from build123d import *
from OCP.BRepFilletAPI import BRepFilletAPI_MakeChamfer

# Parameters (mm, degrees)
SKETCH1_W                = 0.64
SKETCH1_H                = 0.64
BOSS_EXTRUDE1_DEPTH      = 2.05
CUT_EXTRUDE1_DEPTH       = 5
SKETCH3_W                = 1.54
SKETCH3_H                = 0.5
BOSS_EXTRUDE2_DEPTH      = 0.5
BOSS_EXTRUDE3_DEPTH      = 10
BOSS_EXTRUDE3_DEPTH_BACK = 5.05
SKETCH4_W                = 0.64
SKETCH4_H                = 0.64
CHAMFER1_SIZE            = 0.2
CHAMFER1_SIZE2           = 0.115470054
SKETCH5_R                = 0.125
CUT_EXTRUDE2_DEPTH       = 1


with BuildPart() as part:
    # Sketch1 → Boss-Extrude1 (new body)
    with BuildSketch(Plane(origin=(0, 0, 0), x_dir=(1, 0, 0), z_dir=(0, 1, 0))):
        Polygon((-2.04, -1.27), (-0.5, -1.27), (0, -0.77), (0.5, -1.27), (2.04, -1.27), (2.54, -0.77), (2.54, 0.77), (2.04, 1.27), (0.5, 1.27), (0, 0.77), (-0.5, 1.27), (-2.04, 1.27), (-2.54, 0.77), (-2.54, -0.77), align=None)
        with Locations((1.27, 0)):
            Rectangle(SKETCH1_W, SKETCH1_H, mode=Mode.SUBTRACT)
        with Locations((-1.27, 0)):
            Rectangle(SKETCH1_W, SKETCH1_H, mode=Mode.SUBTRACT)
    extrude(amount=-BOSS_EXTRUDE1_DEPTH)

    # Sketch2 → Cut-Extrude1 (cut, symmetric)
    with BuildSketch(Plane.XY):
        Polygon((-2.54, -0.2), (-2.54, 0), (-2.34, 0), align=None)
        Polygon((-0.2, 0), (0.2, 0), (0, -0.2), align=None)
        Polygon((2.34, 0), (2.54, 0), (2.54, -0.2), align=None)
        Polygon((-2.54, -1.85), (-2.34, -2.05), (-2.54, -2.05), align=None)
        Polygon((-0.2, -2.05), (0, -1.85), (0.2, -2.05), align=None)
        Polygon((2.34, -2.05), (2.54, -1.85), (2.54, -2.05), align=None)
    extrude(amount=CUT_EXTRUDE1_DEPTH, both=True, mode=Mode.SUBTRACT)

    # Sketch3 → Boss-Extrude2 (add)
    with BuildSketch(Plane.XZ.offset(2.05)):
        with Locations((-1.27, -1.02)):
            Rectangle(SKETCH3_W, SKETCH3_H)
        with Locations((-1.27, 1.02)):
            Rectangle(SKETCH3_W, SKETCH3_H)
        with Locations((1.27, 1.02)):
            Rectangle(SKETCH3_W, SKETCH3_H)
        with Locations((1.27, -1.02)):
            Rectangle(SKETCH3_W, SKETCH3_H)
    extrude(amount=BOSS_EXTRUDE2_DEPTH)

    # Sketch4 → Boss-Extrude3 (add, two sides: drawn at the far end of the back side and taken through both)
    with BuildSketch(Plane(origin=(0, 0, 0), x_dir=(1, 0, 0), z_dir=(0, 1, 0)).offset(-BOSS_EXTRUDE3_DEPTH_BACK)):
        with Locations((-1.27, 0)):
            Rectangle(SKETCH4_W, SKETCH4_H)
        with Locations((1.27, 0)):
            Rectangle(SKETCH4_W, SKETCH4_H)
    extrude(amount=BOSS_EXTRUDE3_DEPTH + BOSS_EXTRUDE3_DEPTH_BACK)

    # Chamfer1: one chamfer whose edges measure the first distance from different faces: ONE call of the kernel's chamfer builder (chamfer() names one face for all edges)
    chamfer1_edges_1 = [part.edges().sort_by_distance(p)[0] for p in [
        (-1.59, -5.05, 0),
    ]]
    chamfer1_side_1 = [part.faces().sort_by_distance(p)[0] for p in [
        (-1.59, -3.55, 0),
    ]]
    chamfer1_edges_2 = [part.edges().sort_by_distance(p)[0] for p in [
        (-1.27, -5.05, -0.32),
    ]]
    chamfer1_side_2 = [part.faces().sort_by_distance(p)[0] for p in [
        (-1.27, -3.55, -0.32),
    ]]
    chamfer1_edges_3 = [part.edges().sort_by_distance(p)[0] for p in [
        (-0.95, -5.05, 0),
    ]]
    chamfer1_side_3 = [part.faces().sort_by_distance(p)[0] for p in [
        (-0.95, -3.55, 0),
    ]]
    chamfer1_edges_4 = [part.edges().sort_by_distance(p)[0] for p in [
        (-1.27, -5.05, 0.32),
    ]]
    chamfer1_side_4 = [part.faces().sort_by_distance(p)[0] for p in [
        (-1.27, -3.55, 0.32),
    ]]
    chamfer1_edges_5 = [part.edges().sort_by_distance(p)[0] for p in [
        (-1.59, 10, 0),
    ]]
    chamfer1_side_5 = [part.faces().sort_by_distance(p)[0] for p in [
        (-1.59, 5, 0),
    ]]
    chamfer1_edges_6 = [part.edges().sort_by_distance(p)[0] for p in [
        (-1.27, 10, 0.32),
    ]]
    chamfer1_side_6 = [part.faces().sort_by_distance(p)[0] for p in [
        (-1.27, 5, 0.32),
    ]]
    chamfer1_edges_7 = [part.edges().sort_by_distance(p)[0] for p in [
        (-0.95, 10, 0),
    ]]
    chamfer1_side_7 = [part.faces().sort_by_distance(p)[0] for p in [
        (-0.95, 5, 0),
    ]]
    chamfer1_edges_8 = [part.edges().sort_by_distance(p)[0] for p in [
        (-1.27, 10, -0.32),
    ]]
    chamfer1_side_8 = [part.faces().sort_by_distance(p)[0] for p in [
        (-1.27, 5, -0.32),
    ]]
    chamfer1_edges_9 = [part.edges().sort_by_distance(p)[0] for p in [
        (0.95, -5.05, 0),
    ]]
    chamfer1_side_9 = [part.faces().sort_by_distance(p)[0] for p in [
        (0.95, -3.55, 0),
    ]]
    chamfer1_edges_10 = [part.edges().sort_by_distance(p)[0] for p in [
        (1.27, -5.05, -0.32),
    ]]
    chamfer1_side_10 = [part.faces().sort_by_distance(p)[0] for p in [
        (1.27, -3.55, -0.32),
    ]]
    chamfer1_edges_11 = [part.edges().sort_by_distance(p)[0] for p in [
        (1.59, -5.05, 0),
    ]]
    chamfer1_side_11 = [part.faces().sort_by_distance(p)[0] for p in [
        (1.59, -3.55, 0),
    ]]
    chamfer1_edges_12 = [part.edges().sort_by_distance(p)[0] for p in [
        (1.27, -5.05, 0.32),
    ]]
    chamfer1_side_12 = [part.faces().sort_by_distance(p)[0] for p in [
        (1.27, -3.55, 0.32),
    ]]
    chamfer1_edges_13 = [part.edges().sort_by_distance(p)[0] for p in [
        (0.95, 10, 0),
    ]]
    chamfer1_side_13 = [part.faces().sort_by_distance(p)[0] for p in [
        (0.95, 5, 0),
    ]]
    chamfer1_edges_14 = [part.edges().sort_by_distance(p)[0] for p in [
        (1.27, 10, 0.32),
    ]]
    chamfer1_side_14 = [part.faces().sort_by_distance(p)[0] for p in [
        (1.27, 5, 0.32),
    ]]
    chamfer1_edges_15 = [part.edges().sort_by_distance(p)[0] for p in [
        (1.59, 10, 0),
    ]]
    chamfer1_side_15 = [part.faces().sort_by_distance(p)[0] for p in [
        (1.59, 5, 0),
    ]]
    chamfer1_edges_16 = [part.edges().sort_by_distance(p)[0] for p in [
        (1.27, 10, -0.32),
    ]]
    chamfer1_side_16 = [part.faces().sort_by_distance(p)[0] for p in [
        (1.27, 5, -0.32),
    ]]
    chamfer1 = BRepFilletAPI_MakeChamfer(part.part.solid().wrapped)
    for e in chamfer1_edges_1:
        chamfer1.Add(CHAMFER1_SIZE, CHAMFER1_SIZE2, e.wrapped, chamfer1_side_1[0].wrapped)  # the first distance lies on this face
    for e in chamfer1_edges_2:
        chamfer1.Add(CHAMFER1_SIZE, CHAMFER1_SIZE2, e.wrapped, chamfer1_side_2[0].wrapped)  # the first distance lies on this face
    for e in chamfer1_edges_3:
        chamfer1.Add(CHAMFER1_SIZE, CHAMFER1_SIZE2, e.wrapped, chamfer1_side_3[0].wrapped)  # the first distance lies on this face
    for e in chamfer1_edges_4:
        chamfer1.Add(CHAMFER1_SIZE, CHAMFER1_SIZE2, e.wrapped, chamfer1_side_4[0].wrapped)  # the first distance lies on this face
    for e in chamfer1_edges_5:
        chamfer1.Add(CHAMFER1_SIZE, CHAMFER1_SIZE2, e.wrapped, chamfer1_side_5[0].wrapped)  # the first distance lies on this face
    for e in chamfer1_edges_6:
        chamfer1.Add(CHAMFER1_SIZE, CHAMFER1_SIZE2, e.wrapped, chamfer1_side_6[0].wrapped)  # the first distance lies on this face
    for e in chamfer1_edges_7:
        chamfer1.Add(CHAMFER1_SIZE, CHAMFER1_SIZE2, e.wrapped, chamfer1_side_7[0].wrapped)  # the first distance lies on this face
    for e in chamfer1_edges_8:
        chamfer1.Add(CHAMFER1_SIZE, CHAMFER1_SIZE2, e.wrapped, chamfer1_side_8[0].wrapped)  # the first distance lies on this face
    for e in chamfer1_edges_9:
        chamfer1.Add(CHAMFER1_SIZE, CHAMFER1_SIZE2, e.wrapped, chamfer1_side_9[0].wrapped)  # the first distance lies on this face
    for e in chamfer1_edges_10:
        chamfer1.Add(CHAMFER1_SIZE, CHAMFER1_SIZE2, e.wrapped, chamfer1_side_10[0].wrapped)  # the first distance lies on this face
    for e in chamfer1_edges_11:
        chamfer1.Add(CHAMFER1_SIZE, CHAMFER1_SIZE2, e.wrapped, chamfer1_side_11[0].wrapped)  # the first distance lies on this face
    for e in chamfer1_edges_12:
        chamfer1.Add(CHAMFER1_SIZE, CHAMFER1_SIZE2, e.wrapped, chamfer1_side_12[0].wrapped)  # the first distance lies on this face
    for e in chamfer1_edges_13:
        chamfer1.Add(CHAMFER1_SIZE, CHAMFER1_SIZE2, e.wrapped, chamfer1_side_13[0].wrapped)  # the first distance lies on this face
    for e in chamfer1_edges_14:
        chamfer1.Add(CHAMFER1_SIZE, CHAMFER1_SIZE2, e.wrapped, chamfer1_side_14[0].wrapped)  # the first distance lies on this face
    for e in chamfer1_edges_15:
        chamfer1.Add(CHAMFER1_SIZE, CHAMFER1_SIZE2, e.wrapped, chamfer1_side_15[0].wrapped)  # the first distance lies on this face
    for e in chamfer1_edges_16:
        chamfer1.Add(CHAMFER1_SIZE, CHAMFER1_SIZE2, e.wrapped, chamfer1_side_16[0].wrapped)  # the first distance lies on this face
    add(Compound.cast(chamfer1.Shape()), mode=Mode.REPLACE)

    # Sketch5 → Cut-Extrude2 (cut)
    with BuildSketch(Plane.XZ.offset(5.05)):
        with Locations(Location((-1.27, 0, 0), (0, 0, 270))):
            Circle(SKETCH5_R)
    extrude(amount=-CUT_EXTRUDE2_DEPTH, mode=Mode.SUBTRACT)


solid = part.part
Geometry: final body of the model. Coordinates: model frame, mm. Round coordinates to 2 decimals unless told otherwise and drop trailing zeros. Order: outer loops, then holes, each group sorted by start corner. A loop starts at its lowest first (then second) coordinate and runs counter-clockwise, first axis right, second up. Notation, with made-up numbers: (1, 7.5) -> (49, 7.5) arc R20 ccw to (49, 29.5) -> close; hole circle Ø1 at (75.25, 63). An arc over 180 degrees is marked (long way). Put each result on its own line as item: value. Start each with the question number.
Q1. Section C-C on y = -0.5. Return the cut outline in (x, z), and give its area (3 significant figures).
Q2. First-contact query: pin 1 (0.7 mm diameter, centred on x = -1.5, y = -3.5, fed in from +Z); pin 2 (1.5 mm diameter, centred on x = 0, z = -1, fed in from +Y); pin 3 (0.5 mm diameter, centred on y = -3.5, z = 0, fed in from -X). Flat tips, straight axial feed; report the tip coordinate or a pass-through.
Q3. Pull-direction query (X, two-part tool) for faces 1 (the flat face through (2, -2.05, 0)), 2 (the flat face through (-1, -1, 1.27)), 3 (the flat face through (-2.54, -1, 0)); classes: +X half, -X half, draft (parallel to the pull), parting line (faces both ways), or undercut.
Q4. Line query: probe 1 along X at (y, z) = (-4.8, 0) (3 decimals); probe 2 along Y at (x, z) = (-0.6, 0.5); probe 3 along Z at (x, y) = (-1, 7.5). Output: solid intervals per line, ascending.
Q5. Section A-A on z = 1.1. Return the cut outline in (x, y).
Q6. Section B-B on y = -2.75. Return the cut outline in (x, z).
Q7. Section D-D on z = -0.55. Return the cut outline in (x, y).
Ans:
1. outline: (-2.54, -0.77) -> (-2.04, -1.27) -> (-0.5, -1.27) -> (0, -0.77) -> (0.5, -1.27) -> (2.04, -1.27) -> (2.54, -0.77) -> (2.54, 0.77) -> (2.04, 1.27) -> (0.5, 1.27) -> (0, 0.77) -> (-0.5, 1.27) -> (-2.04, 1.27) -> (-2.54, 0.77) -> close
1. area: 11.9 mm2
2. pin 1: stops at z = 0.32
2. pin 2: stops at y = 0
2. pin 3: stops at x = -1.59
3. face 1: undercut
3. face 2: draft
3. face 3: -X half
4. probe 1: x = -1.59 to -1.395, -1.145 to -0.95, 0.95 to 1.59
4. probe 2: y = -2.05 to 0
4. probe 3: z = -0.32 to 0.32
5. outline: (-2.21, -2.05) -> (-2.04, -2.05) -> (-2.04, -2.55) -> (-0.5, -2.55) -> (-0.5, -2.05) -> (-0.33, -2.05) -> (-0.33, 0) -> (-2.21, 0) -> close; (0.33, -2.05) -> (0.5, -2.05) -> (0.5, -2.55) -> (2.04, -2.55) -> (2.04, -2.05) -> (2.21, -2.05) -> (2.21, 0) -> (0.33, 0) -> close
6. outline: (-1.59, -0.32) -> (-0.95, -0.32) -> (-0.95, 0.32) -> (-1.59, 0.32) -> close; (0.95, -0.32) -> (1.59, -0.32) -> (1.59, 0.32) -> (0.95, 0.32) -> close
7. outline: (-2.54, -1.85) -> (-2.34, -2.05) -> (-0.2, -2.05) -> (0, -1.85) -> (0.2, -2.05) -> (2.34, -2.05) -> (2.54, -1.85) -> (2.54, -0.2) -> (2.34, 0) -> (0.2, 0) -> (0, -0.2) -> (-0.2, 0) -> (-2.34, 0) -> (-2.54, -0.2) -> close
